Check sheet for the modelled part. Datum: model origin and axes. Units: mm. Round coordinates to 2 decimals unless told otherwise and drop trailing zeros. Order: outer loops, then holes, each group sorted by start corner. A loop starts at its lowest first (then second) coordinate and runs counter-clockwise, first axis right, second up. Notation, with made-up numbers: (15.25, 43.5) -> (72.25, 43.5) arc R30 cw to (72.25, 79.5) -> close; hole circle Ø10 at (30, -13.75). An arc over 180 degrees is marked (long way). Answer in a Markdown table with one row per item.
from build123d import *

# Parameters (mm, degrees)
SKETCH1_W           = 4
SKETCH1_H           = 3
BOSS_EXTRUDE1_DEPTH = 1.5
SPLIT1_START        = -1.5
SPLIT1_DEPTH        = 3
SPLIT1_2_DEPTH      = 3
SPLIT1_3_DEPTH      = 3
SKETCH5_R           = 0.2
BOSS_EXTRUDE2_DEPTH = 15


# Read off the part's stored shape, not the designer's step: Split1
with BuildPart() as part:
    # Sketch1 → Boss-Extrude1 (new body)
    with BuildSketch(Plane(origin=(0, 0, 0), x_dir=(1, 0, 0), z_dir=(0, 1, 0))):
        Rectangle(SKETCH1_W, SKETCH1_H)
    extrude(amount=BOSS_EXTRUDE1_DEPTH)

    # Split1 outline → Split1 (cut)
    with BuildSketch(Plane.XY.offset(SPLIT1_START)):
        Polygon((-2, 1.5), (-2, 0), (-1.5, 1.5), align=None)
        Polygon((2, 1.5), (1.5, 1.5), (2, 0), align=None)
    extrude(amount=SPLIT1_DEPTH, mode=Mode.SUBTRACT)

    # Sketch5 → Boss-Extrude2 (add)
    with BuildSketch(Plane(origin=(0, 0, -1.5), x_dir=(-1, 0, 0), z_dir=(0, 0, -1))):
        with Locations(Location((0, 0.75, 0), (0, 0, 180))):
            Circle(SKETCH5_R)
        with Locations(Location((-0.875, 0.75, 0), (0, 0, 180))):
            Circle(SKETCH5_R)
        with Locations(Location((0.875, 0.75, 0), (0, 0, 180))):
            Circle(SKETCH5_R)
    extrude(amount=BOSS_EXTRUDE2_DEPTH)


with BuildPart() as body_2:
    # Split1 2 outline → Split1 2 (new body)
    with BuildSketch(Plane.XY.offset(SPLIT1_START)):
        Polygon((-2, 1.5), (-2, 0), (-1.5, 1.5), align=None)
    extrude(amount=SPLIT1_2_DEPTH)


with BuildPart() as body_3:
    # Split1 3 outline → Split1 3 (new body)
    with BuildSketch(Plane.XY.offset(SPLIT1_START)):
        Polygon((2, 1.5), (1.5, 1.5), (2, 0), align=None)
    extrude(amount=SPLIT1_3_DEPTH)


solid = part.part
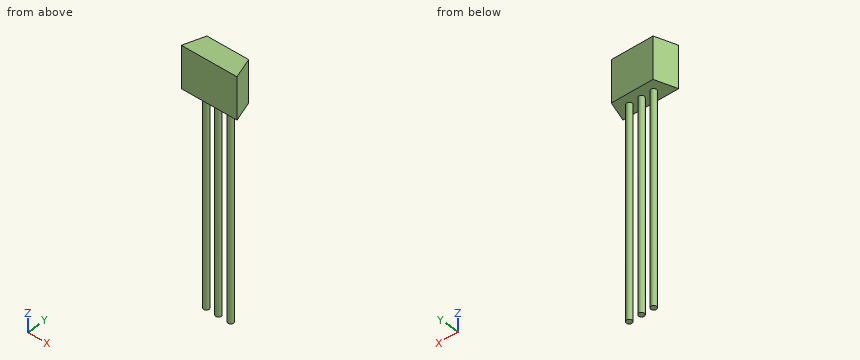
Item 1: Scan lines: line 1 (X direction, y = 0.65, z = -2); line 2 (Z direction, x = 0.45, y = 0.95); line 3 (Y direction, x = 0.85, z = -11). Record each from-to range of solid material in increasing order. Write a range as [from, to].
Result sheet:
| item | result |
|---|---|
| line 1 | x = [-1.05, -0.7], [-0.17, 0.17], [0.7, 1.05] |
| line 2 | z = [-1.5, 1.5] |
| line 3 | y = [0.55, 0.95] |
Item 2: Cross-section at A-A (z = -10). Record the boundary of the cut face in (x, y) (3 decimals), and give its area (3 significant figures).
Result sheet:
| item | result |
|---|---|
| outline | circle Ø0.4 at (-0.875, 0.75); circle Ø0.4 at (0, 0.75); circle Ø0.4 at (0.875, 0.75) |
| area | 0.377 mm^2 |
Item 3: Cross-section at C-C (x = 0). Record the boundary of the cut face in (y, z).
Result sheet:
| item | result |
|---|---|
| outline | (0, -1.5) -> (0.55, -1.5) -> (0.55, -16.5) -> (0.95, -16.5) -> (0.95, -1.5) -> (1.5, -1.5) -> (1.5, 1.5) -> (0, 1.5) -> close |
Item 4: Cross-section at D-D (z = -1). Record the boundary of the cut face in (x, y), and give its area (3 significant figures).
Result sheet:
| item | result |
|---|---|
| outline | (-2, 0) -> (2, 0) -> (1.5, 1.5) -> (-1.5, 1.5) -> close |
| area | 5.25 mm^2 |
Item 5: Cross-section at B-B (y = 0.75). Record the boundary of the cut face in (x, z) (3 decimals).
Result sheet:
| item | result |
|---|---|
| outline | (-1.75, -1.5) -> (-1.075, -1.5) -> (-1.075, -16.5) -> (-0.675, -16.5) -> (-0.675, -1.5) -> (-0.2, -1.5) -> (-0.2, -16.5) -> (0.2, -16.5) -> (0.2, -1.5) -> (0.675, -1.5) -> (0.675, -16.5) -> (1.075, -16.5) -> (1.075, -1.5) -> (1.75, -1.5) -> (1.75, 1.5) -> (-1.75, 1.5) -> close |
